Verification items for the finished model (mm, model axes). Coordinates: 2 decimals unless noted, no trailing zeros. Order: outer loops, then holes, each group sorted by start corner. A loop starts at its lowest first (then second) coordinate and runs counter-clockwise, first axis right, second up. Notation, with made-up numbers: (75, 22.25) -> (86, 22.25) arc R15 cw to (86, 27.25) -> close; hole circle Ø6 at (-4.75, 85.5). An arc over 180 degrees is marked (long way). Use CSV: the item, a comma, the result in double quotes. Start each with the question number.
1) Sectioned sample at B-B on y = 12. Record the boundary of the cut face in (x, z).
2) Sectioned sample at C-C on z = 2.25. Record the boundary of the cut face in (x, y) (1 decimal).
3) Sectioned sample at A-A on x = 93. Record the boundary of the cut face in (y, z), then the cut area to 3 significant figures.
4) Scan lines: line 1 along X through (y, z) = (-16.5, 6); line 2 along Y through (x, z) = (91, -1); line 3 along Y through (x, z) = (36.5, 0.75). Record each from-to range of solid material in increasing order.
5) Go/stop test with flat-tipped pins: pin 1 (1.5 mm diameter, centred on x = 91.5, z = 3.5, fed in from +Y); pin 2 (2 mm diameter, centred on x = -9, z = 4.5, fed in from -Y); pin 3 (3 mm diameter, centred on y = 3.5, z = -1, fed in from -X). Record where each tip stops, or that it passes through.
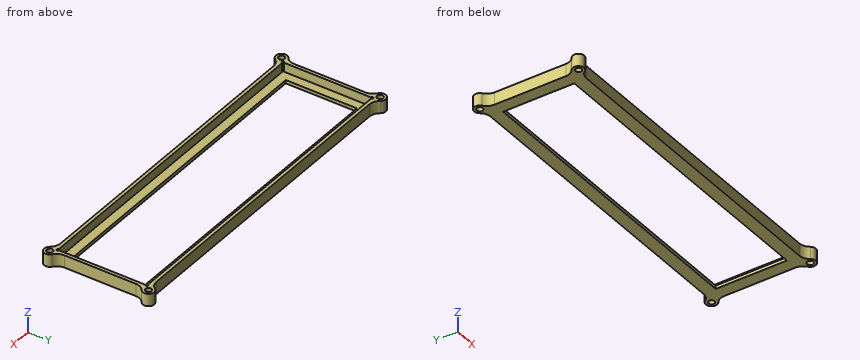
from build123d import *

# Parameters (mm, degrees)
F0_W      = 234.762548
F0_H      = 67.762526
F0_W_2    = 230.000048
F0_H_2    = 63.000026
F1_DEPTH  = 6.35
F2_W      = 234.762548
F2_H      = 67.762526
F2_W_2    = 217.300048
F2_H_2    = 50.300026
F3_DEPTH  = 2.38125
F4_R      = 3.96875
F5_DEPTH  = 8.73125
F6_R      = 7.9375
F7_R      = 2.15265
F8_DEPTH  = 8.73125
F9_R      = 0.79375
F10_DEPTH = 6.35


with BuildPart() as f1:
    # F0 (on Top) → F1 (new body)
    with BuildSketch(Plane.XY):
        Rectangle(F0_W, F0_H)
        Rectangle(F0_W_2, F0_H_2, mode=Mode.SUBTRACT)
    extrude(amount=F1_DEPTH)

    # F2 (on face) → F3 (join)
    with BuildSketch(Plane(origin=(0, 0, 0), x_dir=(1, 0, 0), z_dir=(0, 0, -1))):
        Rectangle(F2_W, F2_H)
        Rectangle(F2_W_2, F2_H_2, mode=Mode.SUBTRACT)
    extrude(amount=F3_DEPTH)

    # F4 (on face) → F5 (join, through all)
    with BuildSketch(Plane.XY.offset(6.35)):
        with Locations((118.36762, 34.867609)):
            Circle(F4_R)
        with Locations((118.36762, -34.867609)):
            Circle(F4_R)
        with Locations((-118.36762, -34.867609)):
            Circle(F4_R)
        with Locations((-118.36762, 34.867609)):
            Circle(F4_R)
    extrude(amount=-F5_DEPTH)

    # F6
    f6_edges = [f1.edges().sort_by_distance(p)[0] for p in [
        (114.523391, 33.881263, 1.984375),
        (117.381274, 31.02338, 1.984375),
        (117.381274, -31.02338, 1.984375),
        (114.523391, -33.881263, 1.984375),
        (-117.381274, -31.02338, 1.984375),
        (-114.523391, -33.881263, 1.984375),
        (-114.523391, 33.881263, 1.984375),
        (-117.381274, 31.02338, 1.984375),
    ]]
    fillet(f6_edges, radius=F6_R)

    # F7 (on face) → F8 (cut, through all)
    with BuildSketch(Plane.XY.offset(6.35)):
        with Locations((118.36762, 34.867609)):
            Circle(F7_R)
        with Locations((118.36762, -34.867609)):
            Circle(F7_R)
        with Locations((-118.36762, 34.867609)):
            Circle(F7_R)
        with Locations((-118.36762, -34.867609)):
            Circle(F7_R)
    extrude(amount=-F8_DEPTH, mode=Mode.SUBTRACT)

    # F9 (on face) → F10 (cut, through all)
    with BuildSketch(Plane.XY.offset(6.35)):
        with Locations((-115.000024, 31.500013)):
            Circle(F9_R)
        with Locations((-115.000024, -31.500013)):
            Circle(F9_R)
        with Locations((115.000024, -31.500013)):
            Circle(F9_R)
        with Locations((115.000024, 31.500013)):
            Circle(F9_R)
    extrude(amount=-F10_DEPTH, mode=Mode.SUBTRACT)


solid = f1.part
Answers follow:
1,outline,"(-117.38, -2.38) -> (-108.65, -2.38) -> (-108.65, 0) -> (-115, 0) -> (-115, 6.35) -> (-117.38, 6.35) -> close; (108.65, -2.38) -> (117.38, -2.38) -> (117.38, 6.35) -> (115, 6.35) -> (115, 0) -> (108.65, 0) -> close"
2,outline,"(-120.7, -31.6) arc R4 ccw (long way) to (-115.1, -37.2) arc R7.9 cw to (-108.7, -33.9) -> (108.7, -33.9) arc R7.9 cw to (115.1, -37.2) arc R4 ccw (long way) to (120.7, -31.6) arc R7.9 cw to (117.4, -25.2) -> (117.4, 25.2) arc R7.9 cw to (120.7, 31.6) arc R4 ccw (long way) to (115.1, 37.2) arc R7.9 cw to (108.7, 33.9) -> (-108.7, 33.9) arc R7.9 cw to (-115.1, 37.2) arc R4 ccw (long way) to (-120.7, 31.6) arc R7.9 cw to (-117.4, 25.2) -> (-117.4, -25.2) arc R7.9 cw to start; hole circle Ø4.3 at (-118.4, -34.9); hole circle Ø4.3 at (-118.4, 34.9); hole (-115, -30.7) arc R0.8 ccw (long way) to (-114.2, -31.5) -> (114.2, -31.5) arc R0.8 ccw (long way) to (115, -30.7) -> (115, 30.7) arc R0.8 ccw (long way) to (114.2, 31.5) -> (-114.2, 31.5) arc R0.8 ccw (long way) to (-115, 30.7) -> close; hole circle Ø4.3 at (118.4, -34.9); hole circle Ø4.3 at (118.4, 34.9)"
3,outline,"(-33.88, -2.38) -> (-25.15, -2.38) -> (-25.15, 0) -> (-31.5, 0) -> (-31.5, 6.35) -> (-33.88, 6.35) -> close; (25.15, -2.38) -> (33.88, -2.38) -> (33.88, 6.35) -> (31.5, 6.35) -> (31.5, 0) -> (25.15, 0) -> close"
3,area,"71.8 mm²"
4,line 1,"x = -117.38 to -115, 115 to 117.38"
4,line 2,"y = -33.88 to -25.15, 25.15 to 33.88"
4,line 3,"y = -33.88 to -31.5, 31.5 to 33.88"
5,pin 1,"stops at y = 33.88"
5,pin 2,"stops at y = -33.88"
5,pin 3,"stops at x = -117.38"
